Model file for the job. Use its own axes, mm. A direction names the side the tool comes from. Coordinates: 2 decimals unless noted, no trailing zeros. Write each loop counter-clockwise with the first axis right and the second up, starting at its lowest first coordinate (ties: lowest second). Pieces come first, ordered by that corner, then holes. Notation, with made-up numbers: (74.5, 55.5) - (98.5, 55.5) arc R21 ccw to (98.5, 66.5) - close; hole circle Ø2 at (85, 55.25). An arc over 180 degrees is marked (long way). Put each result on its own line as item: value. Start each with the question number.
1. Drill centre lines: L1, parallel to Y at x = 11.5, z = 9; L2, parallel to X at y = 8.5, z = 2; L3, parallel to X at y = 6.5, z = -1. Where is each one in solid material? Low to high. Write a range as from..to.
2. Which spindle directions (+Z, -Z, +X, -X, +Y, -Y) get a long thin tool onto all of the face, cutting with end or side? Do faces 1 (the face through (-6.209, 6.056, 14.747)), 2 (the face through (-13, 10, 13)). Say none if no direction does.
3. Saw through at B-B, the plane z = 7. Write the cut outline in (x, y), plus the area to 3 significant figures.
4. Saw through at A-A, the plane y = 4. Write the cut outline in (x, z).
5. Saw through at C-C, the plane x = -6.5. Write the cut outline in (y, z), plus the area to 3 significant figures.
6. Pull direction Z, two halves, no side cores. Call faces 3 (the face through (14.747, 6.056, 6.209)), 4 (the face through (0, 0, 0)), 5 (the face through (8.86, 4.93, 28.14)): released by +Z, released by -Z, zero draft, split by the parting line, or undercut.
7. Drop flat-ended pins along their axis: P1, Ø3, axis at y = 7.5, z = -13, coming from the +X side; P2, Ø3, axis at y = 2, z = 20.5, coming from the -X side; P3, Ø2, axis at x = 11, y = 6.5, coming from the +Z side. Give the stop position or say it passes through.
```python
from build123d import *

# Parameters (mm, degrees)
SKETCH1_R           = 29.5
BOSS_EXTRUDE1_DEPTH = 10
CUT_EXTRUDE1_DEPTH  = 8


with BuildPart() as part:
    # Sketch1 → Boss-Extrude1 (new body)
    with BuildSketch(Plane(origin=(0, 0, 0), x_dir=(1, 0, 0), z_dir=(0, 1, 0))):
        with Locations(Location((0, 0, 0), (0, 0, 270))):
            Circle(SKETCH1_R)
    extrude(amount=BOSS_EXTRUDE1_DEPTH)

    # Sketch2 → Cut-Extrude1 (cut)
    with BuildSketch(Plane(origin=(0, 10, 0), x_dir=(1, 0, 0), z_dir=(0, 1, 0))):
        Polygon((12.245869836, 12.245869836), (0, 17.318275205), (-12.245869836, 12.245869836), (-17.318275205, 0), (-12.245869836, -12.245869836), (0, -17.318275205), (12.245869836, -12.245869836), (17.318275205, 0), align=None)
    extrude(amount=-CUT_EXTRUDE1_DEPTH, mode=Mode.SUBTRACT)


solid = part.part
```
Final values:
1. L1: y = 0..2
1. L2: x = -29.43..-16.49, 16.49..29.43
1. L3: x = -29.48..-16.9, 16.9..29.48
2. face 1: +Y
2. face 2: +Z, -Z, +X, -X, +Y
3. outline: (-28.66, 0) - (28.66, 0) - (28.66, 10) - (14.42, 10) - (14.42, 2) - (-14.42, 2) - (-14.42, 10) - (-28.66, 10) - close
3. area: 342 mm²
4. outline: circle Ø59 at (0, 0); hole (-17.32, 0) - (-12.25, -12.25) - (0, -17.32) - (12.25, -12.25) - (17.32, 0) - (12.25, 12.25) - (0, 17.32) - (-12.25, 12.25) - close
5. outline: (0, -28.77) - (10, -28.77) - (10, -14.63) - (2, -14.63) - (2, 14.63) - (10, 14.63) - (10, 28.77) - (0, 28.77) - close
5. area: 341 mm²
6. face 3: undercut
6. face 4: zero draft
6. face 5: split by the parting line
7. P1: stops at x = 27.17
7. P2: stops at x = -22.57
7. P3: stops at z = 27.75
